Work out the finished part from the listing and answer in its coordinate system (mm). Face numbers are marked on the shaded views. A direction names the side the tool comes from. Give positions to 0.01 mm unless a question says otherwise; leave off trailing zeros. Order: outer loops, then holes, each group sorted by start corner. A loop starts at its lowest first (then second) coordinate and runs counter-clockwise, first axis right, second up.
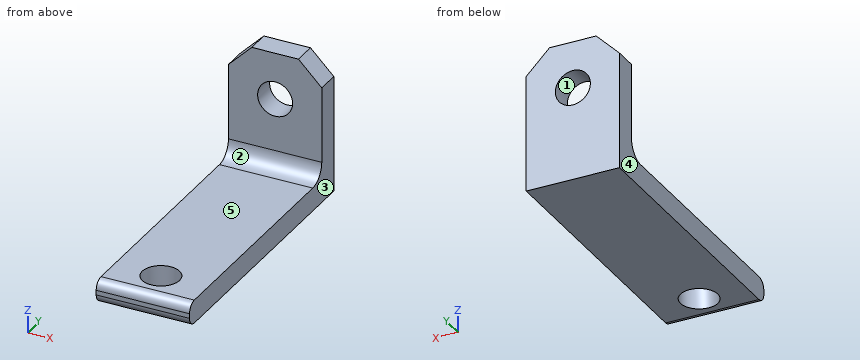
```python
from build123d import *

# Parameters (mm, degrees)
F1_DEPTH = 25.4
F2_R     = 4.7752
F3_R     = 4.7625
F4_DEPTH = 25.4
F5_SIZE  = 6.35
F6_R     = 5.08
F7_DEPTH = 25.4
F8_R     = 2.54


with BuildPart() as f1:
    # F0 (on Right) → F1 (new body)
    with BuildSketch(Plane.YZ):
        Polygon((-76.2, 0), (0, 0), (0, 38.1), (-6.35, 38.1), (-6.35, 6.35), (-76.2, 6.35), align=None)
    extrude(amount=F1_DEPTH)

    # F2
    f2_edges = [f1.edges().sort_by_distance(p)[0] for p in [
        (12.7, -6.35, 6.35),
    ]]
    fillet(f2_edges, radius=F2_R)

    # F3 (on face) → F4 (cut)
    with BuildSketch(Plane(origin=(0, 0, 0), x_dir=(-1, 0, 0), z_dir=(0, 1, 0))):
        with Locations((-12.7, 25.4)):
            Circle(F3_R)
    extrude(amount=-F4_DEPTH, mode=Mode.SUBTRACT)

    # F5
    f5_edges = [f1.edges().sort_by_distance(p)[0] for p in [
        (25.4, -3.175, 38.1),
        (0, -3.175, 38.1),
    ]]
    chamfer(f5_edges, length=F5_SIZE)

    # F6 (on face) → F7 (cut)
    with BuildSketch(Plane(origin=(0, 0, 0), x_dir=(1, 0, 0), z_dir=(0, 0, -1))):
        with Locations((12.7, 66.675)):
            Circle(F6_R)
    extrude(amount=-F7_DEPTH, mode=Mode.SUBTRACT)

    # F8
    f8_edges = [f1.edges().sort_by_distance(p)[0] for p in [
        (12.7, -76.2, 0),
        (12.7, -76.2, 6.35),
    ]]
    fillet(f8_edges, radius=F8_R)


solid = f1.part
```
1. Which of the six approach directions +Z, -Z, +X, -X, +Y, -Y give full straight-line access (tool end or side, diameter ignored) to the marked faces 4 and 5?
Findings below:
face 4: +Z, -Z, -X, +Y, -Y
face 5: +Z, +X, -X, -Y
2. The mould has two halves that part along X. Classify the marked faces 1, 2 and 3: pulls with the +X half, pulls with the -X half, needs draft (parallel to the pull), parting line crosses it, or undercut.
Findings below:
face 1: undercut
face 2: needs draft
face 3: pulls with the +X half
3. The part is cut by section C-C (x = 22). Write down the section's boundary in (y, z).
Findings below:
outline: (-76.2, 2.54) arc R2.54 ccw to (-73.66, 0) - (0, 0) - (0, 35.15) - (-6.35, 35.15) - (-6.35, 11.13) arc R4.78 cw to (-11.13, 6.35) - (-73.66, 6.35) arc R2.54 ccw to (-76.2, 3.81) - close
4. The part is cut by section D-D (y = -23.5). Write down the section's boundary in (x, z), then the cut area to 3 significant figures.
Findings below:
outline: (0, 0) - (25.4, 0) - (25.4, 6.35) - (0, 6.35) - close
area: 161 mm2
5. The part is cut by section A-A (z = 25.4). Write down the section's boundary in (x, y).
Findings below:
outline: (0, -6.35) - (7.94, -6.35) - (7.94, 0) - (0, 0) - close; (17.46, -6.35) - (25.4, -6.35) - (25.4, 0) - (17.46, 0) - close
6. Straight lines are drawn through the part: probe 1 along Z at (x, y) = (12.7, -3.75); probe 2 along X at (y, z) = (-2, 25); probe 3 along Y at (x, z) = (12.7, 2.75) (3 decimals). For each, find the intervals that lie inside material, in ascending order.
Findings below:
probe 1: z = 0 to 20.64, 30.16 to 38.1
probe 2: x = 0 to 7.95, 17.45 to 25.4
probe 3: y = -76.2 to -71.755, -61.595 to 0
7. The part is cut by section B-B (x = 12.7). State how many separate pieces and enclosed holes the cut face has, then the cut area to 3 significant figures.
Findings below:
separate pieces: 3
enclosed holes: 0
area: 563 mm2
8. Given P1, Ø12.5, axis at x = 14.5, y = -34, coming from the +Z side; P2, Ø7.5, axis at x = 18.5, z = 24.5, coming from the -Y side, each flat-ended and moving along its own axis, determine where each tip first touches the part or whether it passes through.
Findings below:
P1: stops at z = 6.35
P2: stops at y = -6.35
